Solid Edge part; units mm, degrees
sketch "Sketch1" plane through (0, 0, 0) normal (0, -1, 0) x (1, 0, 0)
  line L0 (18.5, -10) -> (18.5, 10)
  line L1 (18.5, 10) -> (-18.5, 10)
  line L2 (-18.5, 10) -> (-18.5, -10)
  line L3 (-18.5, -10) -> (18.5, -10)
  circle A0 centre (0, 0) radius 5.25
extrude "Protrusion1" add sketch "Sketch1" against normal blind 2
sketch "Sketch2" plane through (-18.5, 1, 0) normal (-1, 0, 0) x (0, 0, 1)
  line L0 (10, 44) -> (10, -1)
  line L1 (10, -1) -> (-10, -1)
  line L2 (-10, -1) -> (-10, 44)
  line L3 (-10, 44) -> (10, 44)
  circle A0 centre (0, 44) radius 5
extrude "Extrusionsausprägung_2" add sketch "Sketch2" along normal blind 2
chamfer "Fase_1" distance 5 angle 45 1 edges at (-19.5, 45, 10)
chamfer "Fase_2" distance 5 angle 45 1 edges at (-19.5, 45, -10)
sketch "Sketch3" plane through (18.5, 1, 0) normal (1, 0, 0) x (0, 0, -1)
  line L0 (10, -1) -> (10, 44)
  line L1 (10, 44) -> (-10, 44)
  circle A0 centre (0, 44) radius 5
  line L2 (-10, 44) -> (-10, -1)
  line L3 (-10, -1) -> (10, -1)
extrude "Extrusionsausprägung_3" add sketch "Sketch3" along normal blind 2
sketch "Sketch4" plane through (-20.5, 17.5, 0) normal (-1, 0, 0) x (0, 0, 1)
  circle A0 centre (0, 27.5) radius 1.5
extrude "Extrusionsausschnitt_1" cut sketch "Sketch4" against normal blind 41
fillet "Verrundung_1" radius 8 1 edges at (18.5, 2, 0)
fillet "Verrundung_2" radius 8 1 edges at (-18.5, 2, 0)
chamfer "Fase_3" distance 5 angle 45 2 edges at (19.5, 45, -10) (19.5, 45, 10)
sketch "Sketch5" plane through (-0.5, 2, 0) normal (0, 1, 0) x (0, 0, -1)
  circle A0 centre (0, -0.5) radius 7.5
extrude "Extrusionsausprägung_4" add sketch "Sketch5" along normal blind 6
sketch "Sketch6" plane through (-0.5, 2, 0) normal (0, 1, 0) x (0, 0, -1)
  circle A0 centre (0, -0.5) radius 5.1
extrude "Extrusionsausschnitt_2" cut sketch "Sketch6" along normal blind 4
sketch "Sketch7" plane through (0, 8, 0) normal (0, 1, 0) x (-1, 0, 0)
  circle A0 centre (0, 0) radius 4
extrude "Extrusionsausschnitt_3" cut sketch "Sketch7" against normal blind 2
chamfer "Fase_4" distance 2 angle 45 1 edges at (4, 6, 0)
Geometry: final body of the model. Coordinates: model frame, mm. A direction names the side the tool comes from. Give positions to 0.01 mm unless a question says otherwise; leave off trailing zeros. Write each loop counter-clockwise with the first axis right and the second up, starting at its lowest first coordinate (ties: lowest second). Pieces come first, ordered by that corner, then holes. Notation, with made-up numbers: (-23.5, 83) -> (16.5, 83) arc R12 ccw to (16.5, 104) -> close; hole circle Ø5 at (84, -19). An arc over 180 degrees is marked (long way). Answer as a JSON object with one key per item and string values.
1. Ray query, probe 1 along X at (y, z) = (24.5, -7); probe 2 along X at (y, z) = (4.45, 0); probe 3 along Z at (x, y) = (0, 4.9). Return the intervals inside material, ascending. Write a range as from..to.
Ans:
{"probe 1": "x = -20.5..-18.5, 18.5..20.5", "probe 2": "x = -20.5..-16.26, -7.5..-5.1, 5.1..7.5, 16.26..20.5", "probe 3": "z = -7.5..-5.1, 5.1..7.5"}
2. Cut plane D-D on z = -6.5. Output: boundary loops of the cut face in (x, y), and give its area (3 significant figures).
Ans:
{"outline": "(-20.5, 0) -> (20.5, 0) -> (20.5, 43.5) -> (18.5, 43.5) -> (18.5, 10) arc R8 cw to (10.5, 2) -> (3.74, 2) -> (3.74, 8) -> (-3.74, 8) -> (-3.74, 2) -> (-10.5, 2) arc R8 cw to (-18.5, 10) -> (-18.5, 43.5) -> (-20.5, 43.5) -> close", "area": "320 mm^2"}
3. Access query for faces 1 (the flat face through (5, 2, 7)), 2 (the cylindrical face through (-4.5, 4.4, -2.4)), 3 (the flat face through (-20, 43, 7)), 4 (the flat face through (18.5, 30, 0)). Directions: +Z, -Z, +X, -X, +Y, -Y. A direction counts if a zero-diameter tool reaches every point of the face in a straight line with its end or side. Return the directions, or none.
Ans:
{"face 1": "+Y", "face 2": "-Y", "face 3": "+Z, +X, -X, +Y", "face 4": "+Z, -Z, +Y"}
4. Mould query, pull axis Z, two halves, no side actions, for faces 5 (the cylindrical face through (-16.094, 4.281, -0.14)), 6 (the flat face through (0, 1, 10)), 7 (the cylindrical face through (5, 1, 1.6)). Classes: pulls with the +Z half, pulls with the -Z half, needs draft (parallel to the pull), parting line crosses it, or undercut.
Ans:
{"face 5": "needs draft", "face 6": "pulls with the +Z half", "face 7": "undercut"}
5. Cut plane A-A on z = 0. Count the separate pieces of the cut face and the enclosed holes in it, and give its area (3 significant figures).
Ans:
{"separate pieces": "4", "enclosed holes": "0", "area": "298 mm^2"}
6. Cut plane C-C on y = 19.5. Output: boundary loops of the cut face in (x, z), and give its area (3 significant figures).
Ans:
{"outline": "(-20.5, -10) -> (-18.5, -10) -> (-18.5, 10) -> (-20.5, 10) -> close; (18.5, -10) -> (20.5, -10) -> (20.5, 10) -> (18.5, 10) -> close", "area": "80.0 mm^2"}
7. Cut plane B-B on x = 0. Output: boundary loops of the cut face in (y, z).
Ans:
{"outline": "(0, -10) -> (2, -10) -> (2, -7.5) -> (8, -7.5) -> (8, -4) -> (6.9, -5.1) -> (2, -5.1) -> (2, -5.25) -> (0, -5.25) -> close; (0, 5.25) -> (2, 5.25) -> (2, 5.1) -> (6.9, 5.1) -> (8, 4) -> (8, 7.5) -> (2, 7.5) -> (2, 10) -> (0, 10) -> close"}
8. Contact query for flat-ended pins moving along their axis: pin 1 (9 mm diameter, centred on x = 0, z = 0, fed in from +Y); pin 2 (6 mm diameter, centred on x = -1.5, y = 9.5, fed in from +Z). Output: stop coordinate, or through.
Ans:
{"pin 1": "stops at y = 8", "pin 2": "stops at z = 7.5"}
